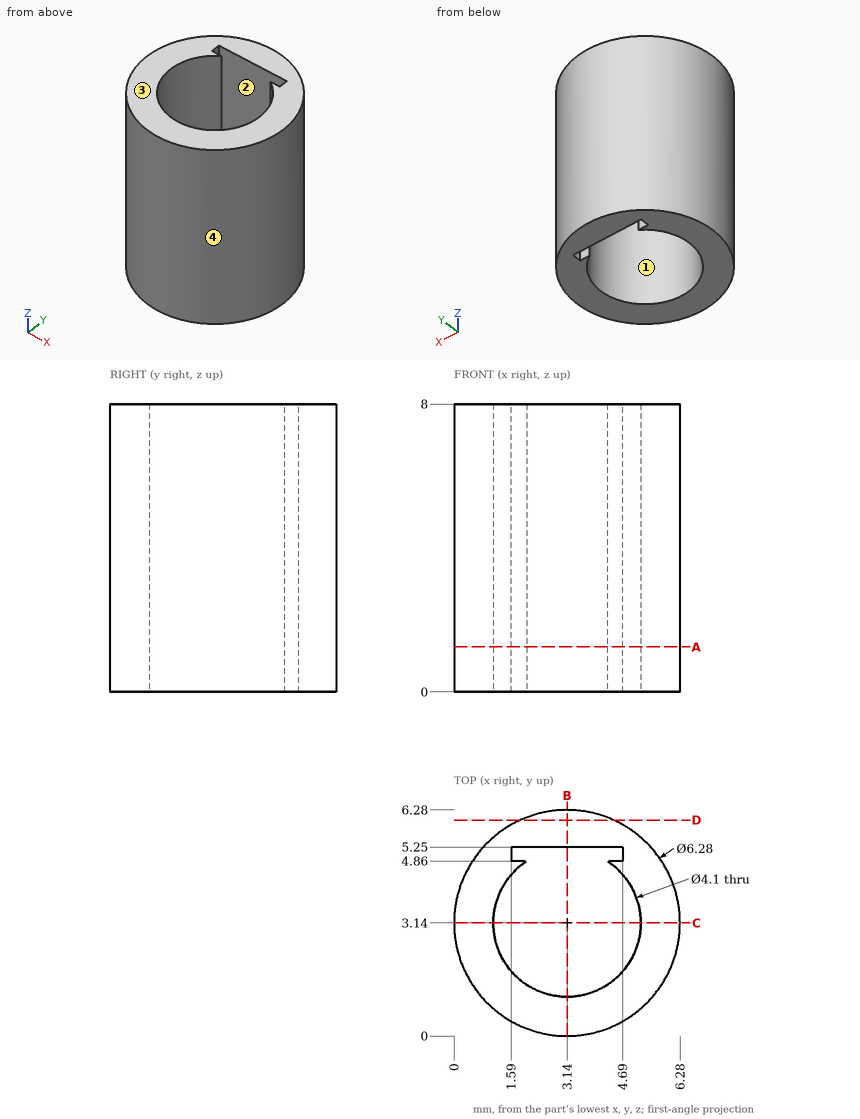
Geometry: see drawing. Coordinates: mm, zero at the bounding-box minimum. Coordinates: 2 decimals unless noted, no trailing zeros. Order: outer loops, then holes, each group sorted by start corner. A loop starts at its lowest first (then second) coordinate and runs counter-clockwise, first axis right, second up. Notation, with made-up numbers: (29.25, -15) - (54.25, -15) arc R14 cw to (54.25, -5) - close; hole circle Ø9 at (-34.75, 46). An arc over 180 degrees is marked (long way). Write each question's results on one line, items separated by ' | '.
1) Section B-B, the plane x = 3.14. Return loops of the section in (y, z), plus the area to 3 significant figures.
Results list:
outline: (0, 0) - (1.09, 0) - (1.09, 8) - (0, 8) - close; (5.25, 0) - (6.28, 0) - (6.28, 8) - (5.25, 8) - close | area: 17.0 mm^2
2) Section D-D, the plane y = 6. Return loops of the section in (x, z).
Results list:
outline: (1.84, 0) - (4.44, 0) - (4.44, 8) - (1.84, 8) - close
3) Pin query (flat end, axial travel): pin 1 (0.5 mm diameter, centred on x = 4.5, z = 5.5, fed in from +Y); pin 2 (1 mm diameter, centred on y = 5.5, z = 2.5, fed in from -X); pin 3 (3 mm diameter, centred on x = 1, z = 5, fed in from -Y); pin 4 (3.5 mm diameter, centred on x = 3, z = 5.5, fed in from -Y). Return the tip coordinate at first contact, or that it passes through.
Results list:
pin 1: y = 6.08 | pin 2: x = 0.61 | pin 3: y = 0.07 | pin 4: y = 0
4) Section A-A, the plane z = 1.25. Return loops of the section in (x, y), plus the area to 3 significant figures.
Results list:
outline: circle Ø6.28 at (3.14, 3.14); hole (1.59, 4.86) - (2.02, 4.86) arc R2.05 ccw (long way) to (4.26, 4.86) - (4.69, 4.86) - (4.69, 5.25) - (1.59, 5.25) - close | area: 17.1 mm^2
5) Section C-C, the plane y = 3.14. Return loops of the section in (x, z), plus the area to 3 significant figures.
Results list:
outline: (0, 0) - (1.09, 0) - (1.09, 8) - (0, 8) - close; (5.19, 0) - (6.28, 0) - (6.28, 8) - (5.19, 8) - close | area: 17.4 mm^2
6) Line query: line 1 (Y direction, x = 3.14, z = 1.75); line 2 (Y direction, x = 1.75, z = 1); line 3 (X direction, y = 3.5, z = 4). Output: solid intervals per line, ascending. Write a range as from..to.
Results list:
line 1: 0..1.09, 5.25..6.28 | line 2: 0.32..1.63, 4.65..4.86, 5.25..5.96 | line 3: 0.02..1.12, 5.16..6.26
7) Pull-direction query (X, two-part tool) for the marked faces 1, 2, 3 and 4; classes: pulls with the +X half, pulls with the -X half, needs draft (parallel to the pull), parting line crosses it, or undercut.
Results list:
face 1: undercut | face 2: undercut | face 3: needs draft | face 4: parting line crosses it
